from build123d import *

# Parameters (mm, degrees)
SKETCH1_W                = 330
SKETCH1_H                = 192
BOSS_EXTRUDE1_DEPTH      = 6
CUT_EXTRUDE1_DEPTH       = 382.837661841
CUT_EXTRUDE1_DEPTH_BACK  = 382.837661841
SKETCH2_R                = 1.5
SKETCH3_R                = 41
CUT_EXTRUDE2_DEPTH       = 382.837661841
CUT_EXTRUDE5_DEPTH       = 10
SKETCH11_R               = 2
CUT_EXTRUDE6_DEPTH       = 10
M5_CLEARANCE_HOLE1_D     = 5.3
M5_CLEARANCE_HOLE1_DEPTH = 11.94
M5_CLEARANCE_HOLE1_TIP   = 1.59228064
CUT_EXTRUDE10_DEPTH      = 382.837661841


with BuildPart() as part:
    # Sketch1 → Boss-Extrude1 (new body)
    with BuildSketch(Plane(origin=(0, 0, 0), x_dir=(1, 0, 0), z_dir=(0, 1, 0))):
        with Locations((165, 96)):
            Rectangle(SKETCH1_W, SKETCH1_H)
    extrude(amount=BOSS_EXTRUDE1_DEPTH)

    # Sketch2 → Cut-Extrude1 (cut, two sides: drawn at the far end of the back side and taken through both)
    with BuildSketch(Plane(origin=(0, 6, 0), x_dir=(1, 0, 0), z_dir=(0, 1, 0)).offset(-CUT_EXTRUDE1_DEPTH_BACK)):
        with Locations(Location((165, 141.5, 0), (0, 0, 270))):
            Circle(SKETCH2_R)
        with Locations(Location((197.173358544, 128.173358544, 0), (0, 0, 270))):
            Circle(SKETCH2_R)
        with Locations(Location((210.5, 96, 0), (0, 0, 270))):
            Circle(SKETCH2_R)
        with Locations(Location((165, 50.5, 0), (0, 0, 270))):
            Circle(SKETCH2_R)
        with Locations(Location((132.826641456, 63.826641456, 0), (0, 0, 270))):
            Circle(SKETCH2_R)
        with Locations(Location((119.5, 96, 0), (0, 0, 270))):
            Circle(SKETCH2_R)
        with Locations(Location((132.826641456, 128.173358544, 0), (0, 0, 270))):
            Circle(SKETCH2_R)
        with Locations(Location((197.173358544, 63.826641456, 0), (0, 0, 270))):
            Circle(SKETCH2_R)
    extrude(amount=CUT_EXTRUDE1_DEPTH + CUT_EXTRUDE1_DEPTH_BACK, mode=Mode.SUBTRACT)

    # Sketch3 → Cut-Extrude2 (cut, through all)
    with BuildSketch(Plane(origin=(0, 6, 0), x_dir=(1, 0, 0), z_dir=(0, 1, 0))):
        with Locations(Location((165, 96, 0), (0, 0, 270))):
            Circle(SKETCH3_R)
    extrude(amount=-CUT_EXTRUDE2_DEPTH, mode=Mode.SUBTRACT)

    # Sketch10 → Cut-Extrude5 (cut)
    with BuildSketch(Plane.XZ):
        with BuildLine():
            Line((123, -136.8), (115, -136.8))
            ThreePointArc((115, -136.8), (111.8, -140), (115, -143.2))
            Line((115, -143.2), (123, -143.2))
            ThreePointArc((123, -143.2), (126.2, -140), (123, -136.8))
        make_face()
        with BuildLine():
            Line((73, -136.8), (65, -136.8))
            ThreePointArc((65, -136.8), (61.8, -140), (65, -143.2))
            Line((65, -143.2), (73, -143.2))
            ThreePointArc((73, -143.2), (76.2, -140), (73, -136.8))
        make_face()
        with BuildLine():
            Line((73, -86.8), (65, -86.8))
            ThreePointArc((65, -86.8), (61.8, -90), (65, -93.2))
            Line((65, -93.2), (73, -93.2))
            ThreePointArc((73, -93.2), (76.2, -90), (73, -86.8))
        make_face()
    extrude(amount=-CUT_EXTRUDE5_DEPTH, mode=Mode.SUBTRACT)

    # Sketch11 → Cut-Extrude6 (cut)
    with BuildSketch(Plane.XZ):
        with Locations(Location((125, -56, 0), (0, 0, 270))):
            Circle(SKETCH11_R)
        with Locations(Location((205, -56, 0), (0, 0, 270))):
            Circle(SKETCH11_R)
        with Locations(Location((205, -136, 0), (0, 0, 270))):
            Circle(SKETCH11_R)
    extrude(amount=-CUT_EXTRUDE6_DEPTH, mode=Mode.SUBTRACT)

    # M5 Clearance Hole1
    with Locations(Plane(origin=(0, 6, 0), x_dir=(1, 0, 0), z_dir=(0, 1, 0))):
        with Locations((10, 172), (10, 10), (320, 10), (320, 172)):
            Hole(M5_CLEARANCE_HOLE1_D / 2, depth=M5_CLEARANCE_HOLE1_DEPTH)
            with Locations((0, 0, -(M5_CLEARANCE_HOLE1_DEPTH + M5_CLEARANCE_HOLE1_TIP / 2))):  # 118° drill point
                Cone(0, M5_CLEARANCE_HOLE1_D / 2, M5_CLEARANCE_HOLE1_TIP, mode=Mode.SUBTRACT)

    # Sketch19 → Cut-Extrude10 (cut, through all)
    with BuildSketch(Plane(origin=(0, 6, 0), x_dir=(1, 0, 0), z_dir=(0, 1, 0))):
        with BuildLine():
            Line((25, 131), (25, 61))
            ThreePointArc((25, 61), (0, 36), (-25, 61))
            Line((-25, 61), (-25, 131))
            ThreePointArc((-25, 131), (0, 156), (25, 131))
        make_face()
        with BuildLine():
            Line((305, 131), (305, 61))
            ThreePointArc((305, 61), (330, 36), (355, 61))
            Line((355, 61), (355, 131))
            ThreePointArc((355, 131), (330, 156), (305, 131))
        make_face()
    extrude(amount=-CUT_EXTRUDE10_DEPTH, mode=Mode.SUBTRACT)


solid = part.part
Model file for the job. Use its own axes, mm. A direction names the side the tool comes from. Coordinates: 2 decimals unless noted, no trailing zeros. Order: outer loops, then holes, each group sorted by start corner. A loop starts at its lowest first (then second) coordinate and runs counter-clockwise, first axis right, second up. Notation, with made-up numbers: (44, 41) -> (77, 41) arc R25 ccw to (77, 53) -> close; hole circle Ø4 at (33, 33). An arc over 180 degrees is marked (long way). Return JSON: item names as keys, results as strings. Group by question number.
Item 1: Tool access for faces 4 (the flat face through (25, 3, -96)), 5 (the flat face through (69, 3, -136.8)), 6 (the cylindrical face through (312.129, 3.042, -43.518)): list every direction of +Z, -Z, +X, -X, +Y, -Y with a clear straight run to the whole face (end or side of a thin tool).
Item 2: Saw through at A-A on z = -112. Write the cut outline in (x, y).
Item 3: Saw through at C-C on z = -45.5. Write the cut outline in (x, y), then the cut area to 3 significant figures.
Item 4: Saw through at B-B on y = 2.8. State how many separate pieces and enclosed holes the cut face has, then the cut area to 3 significant figures.
Item 5: Wall check: line 1 along X through (y, z) = (4.85, -96); line 2 along X through (y, z) = (3.15, -141); line 3 along Z through (x, y) = (10, 3.5). Give the ranges that are in metal, low to high. Write a range as [from, to].
Item 6: Pull direction Z, two halves, no side cores. Call faces 1 (the flat face through (330, 3, -18)), 2 (the cylindrical face through (126.2, 3, -140.1)), 3 (the flat face through (163, 3, -192)): pulls with the +Z half, pulls with the -Z half, needs draft (parallel to the pull), parting line crosses it, or undercut.
Item 7: Flat gauge pin, fed straight in: P1, Ø1, axis at y = 3, z = -83, coming from the -X side. Where does the tip first touch, or does it go through?
Values found:
{
 "1": {"face 4": "-X, +Y, -Y", "face 5": "+Y, -Y", "face 6": "+X, +Y, -Y"},
 "2": {"outline": "(25, 0) -> (127.25, 0) -> (127.25, 6) -> (25, 6) -> close; (202.75, 0) -> (305, 0) -> (305, 6) -> (202.75, 6) -> close"},
 "3": {"outline": "(19.62, 0) -> (310.38, 0) -> (310.38, 6) -> (19.62, 6) -> close", "area": "1,740 mm2"},
 "4": {"separate pieces": "1", "enclosed holes": "19", "area": "52,200 mm2"},
 "5": {"line 1": "x = [25, 118], [121, 124], [206, 209], [212, 305]", "line 2": "x = [22.91, 61.96], [76.04, 111.96], [126.04, 163.59], [166.41, 307.09]", "line 3": "z = [-192, -174.65], [-169.35, -153.91], [-38.09, -12.65], [-7.35, 0]"},
 "6": {"face 1": "needs draft", "face 2": "undercut", "face 3": "pulls with the -Z half"},
 "7": {"P1": "stops at x = 25"}
}
